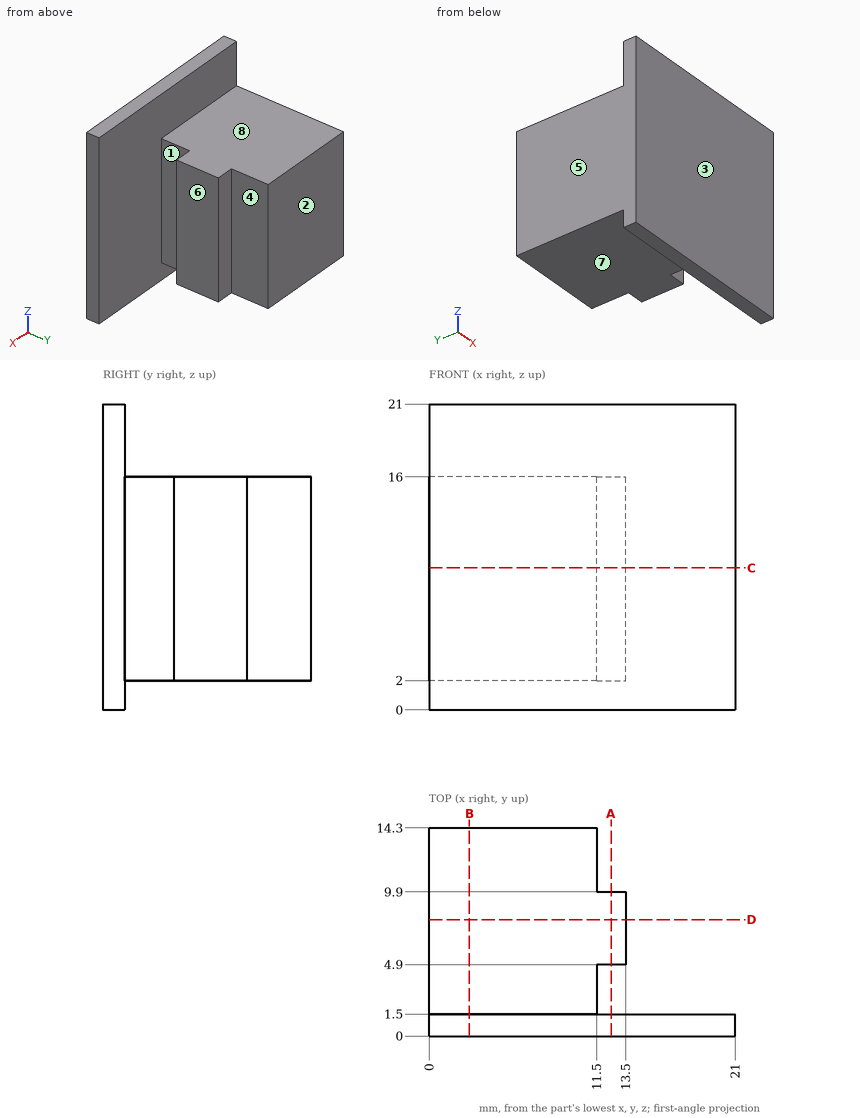
Design review of the part shown in the three views and the two pictorial views. Dimensions are in mm from the part's minimum x, y and z. A direction names the side the tool comes from. Round coordinates to 2 decimals unless told otherwise and drop trailing zeros. Write each loop counter-clockwise with the first axis right and the second up, starting at its lowest first coordinate (ties: lowest second). Pieces come first, ordered by that corner, then holes.
Item 1: We need section C-C on z = 9.75. Write out the cut boundary in (x, y).
Item 2: We need section A-A on x = 12.5. Write out the cut boundary in (y, z), and give its area (4 significant figures).
Item 3: We need section B-B on x = 2.75. Write out the cut boundary in (y, z), and give its area (3 significant figures).
Item 4: Clearance check with flat-ended pins moving along their axes: pin 1 Ø6.5 at (x, y) = (9, 8) entering from +Z; pin 2 Ø1.3 at (y, z) = (12, 8.5) entering from +X; pin 3 Ø8 at (y, z) = (9.5, 10.5) entering from +X; pin 4 Ø6 at (x, y) = (17, 11) entering from -Z. State where each tip first meets the part, or that it passes through.
Item 5: For the marked faces 5, 6, 7 and 8, list the 3-axis set-ups (+Z, -Z, +X, -X, +Y, -Y) from which the entire face can be reached by the end or side of a thin tool; tool diameter is ignored.
Item 6: For probe 1 along Y at (x, z) = (12, 11.75); probe 2 along X at (y, z) = (5.75, 4.25); probe 3 along Z at (x, y) = (10.75, 13), list the stretches that pass through material, from the lowest coordinate up.
Item 7: We need section D-D on y = 8. Write out the cut boundary in (x, z), and give its area (3 significant figures).
Item 8: The part is to be moulded in two halves that separate along Y. For the marked faces 1, 2, 3 and 4, say which applies: +Y half, -Y half, draft (parallel to the pull), parting line (faces both ways), or undercut.
Returned:
1. outline: (0, 0) - (21, 0) - (21, 1.5) - (11.5, 1.5) - (11.5, 4.9) - (13.5, 4.9) - (13.5, 9.9) - (11.5, 9.9) - (11.5, 14.3) - (0, 14.3) - close
2. outline: (0, 0) - (1.5, 0) - (1.5, 21) - (0, 21) - close; (4.9, 2) - (9.9, 2) - (9.9, 16) - (4.9, 16) - close
2. area: 101.5 mm2
3. outline: (0, 0) - (1.5, 0) - (1.5, 2) - (14.3, 2) - (14.3, 16) - (1.5, 16) - (1.5, 21) - (0, 21) - close
3. area: 211 mm2
4. pin 1: stops at z = 16
4. pin 2: stops at x = 11.5
4. pin 3: stops at x = 13.5
4. pin 4: passes through
5. face 5: +Z, -Z, -X, +Y, -Y
5. face 6: +Z, -Z, +X, +Y
5. face 7: -Z, +X, -X, +Y
5. face 8: +Z, +X, -X, +Y
6. probe 1: y = 0 to 1.5, 4.9 to 9.9
6. probe 2: x = 0 to 13.5
6. probe 3: z = 2 to 16
7. outline: (0, 2) - (13.5, 2) - (13.5, 16) - (0, 16) - close
7. area: 189 mm2
8. face 1: undercut
8. face 2: +Y half
8. face 3: -Y half
8. face 4: draft
